The model under review builds one solid part; all positions refer to its coordinate system, in mm. A direction names the side the tool comes from. Coordinates: 2 decimals unless noted, no trailing zeros. Order: outer loops, then holes, each group sorted by start corner. A loop starts at its lowest first (then second) coordinate and runs counter-clockwise, first axis right, second up.
Autodesk Inventor part; units mm, degrees
ref_plane "YZ Plane" through (0, 0, 0) normal (1, 0, 0) x (0, 1, 0)
ref_plane "XZ Plane" through (0, 0, 0) normal (0, 1, 0) x (-1, 0, 0)
ref_plane "XY Plane" through (0, 0, 0) normal (0, 0, 1) x (1, 0, 0)
sketch "sketch" plane through (0, 0, 0) normal (0, 0, 1) x (1, 0, 0)
  line L0 (-10.4, 0) -> (62.4, 0) construction
  line L1 (0, -8.8) -> (0, 31.8) construction
  line L2 (0, 26) -> (52, 26)
  line L3 (52, 26) -> (52, 0)
  line L4 (52, 0) -> (0, 0)
  line L5 (0, 0) -> (0, 26)
  circle A0 centre (3.5, 19) radius 1.5
  circle A1 centre (3.5, 10) radius 1.5
  circle A2 centre (48.5, 19) radius 1.5
  circle A3 centre (48.5, 10) radius 1.5
  line L6 (10, 23) -> (42, 23)
  line L7 (42, 23) -> (42, 0)
  line L8 (42, 0) -> (10, 0)
  line L9 (10, 0) -> (10, 23)
  line L10 (0, 0) -> (52, 0)
  line L11 (52, 0) -> (52, -3)
  line L12 (52, -3) -> (0, -3)
  line L13 (0, -3) -> (0, 0)
  line L14 (7, 23) -> (10, 23)
  line L15 (10, 23) -> (10, 0)
  line L16 (10, 0) -> (7, 0)
  line L17 (7, 0) -> (7, 23)
  line L18 (42, 23) -> (45, 23)
  line L19 (45, 23) -> (45, 0)
  line L20 (45, 0) -> (42, 0)
  line L21 (42, 0) -> (42, 23)
  line L22 (0, 23) -> (7, 23)
  line L23 (45, 23) -> (52, 23)
  line L24 (7, 26) -> (7, 22.7671)
  line L25 (45, 26) -> (45, 23)
  line L26 (7, 0) -> (7, -3)
  line L27 (45, 0) -> (45, -3)
  point P0 (52, 0)
  dimension "d0" = 26
  dimension "d1" = 52
  dimension "d2" = 3
  dimension "d3" = 3
  dimension "d4" = 3
  dimension "d5" = 3
  dimension "d6" = 3.5
  dimension "d7" = 3.5
  dimension "d8" = 3.5
  dimension "d10" = 7
  dimension "d11" = 7
  dimension "d12" = 10
  dimension "d13" = 10
  dimension "d14" = 3
  dimension "d15" = 10
  dimension "d16" = 10
  dimension "d17" = 3
  dimension "d18" = 3
  dimension "d19" = 3
  dimension "d20" = 3.5
extrude "body" add sketch "sketch" along normal blind 50 contours L2 L25 L18 L6 L14 L24 | L14 L9 L4 L17 | L19 L4 L7 L18 | L4 L27 L12 L26
extrude "bolt" add sketch "sketch" along normal blind 1.5 contours L2 L24 L22 L5 | L22 L17 L4 L5 | L2 L3 L23 L25 | L4 L26 L12 L13 | L23 L3 L4 L19 | L4 L11 L12 L27
equation "\"d3\" = d2"
equation "\"d4\" = d2"
equation "\"d5\" = d2"
equation "\"d7\" = d6"
equation "\"d8\" = d6"
equation "\"d11\" = d10"
equation "\"d13\" = d12"
properties part number "battery"
(1) Consider section D-D (y = 19). Give the boundary of the cut face in (x, z), then the cut area to 3 significant figures.
(2) Consider section A-A (y = 16). Give the boundary of the cut face in (x, z), then the cut area to 3 significant figures.
(3) The part is to be moulded in two halves that separate along Y. For faces 1 (the face through (26, 0, 25)), 2 (the face through (45, 12, 25)), 3 (the face through (26, 26, 25)), say which applies: +Y half, -Y half, draft (parallel to the pull), parting line (faces both ways), or undercut.
(4) Tool access review of faces 4 (the face through (7, 12, 25)), 5 (the face through (48, 12, 1.5)), 6 (the face through (10, 11, 25)), 7 (the face through (26, -1, 50)): name each direction out of +Z, -Z, +X, -X, +Y, -Y from which nothing blocks a thin tool from reaching the whole face with its end or side.
(5) Wall thickness on line 1 (X direction, y = 11.5, z = 14); line 2 (Y direction, x = 25, z = 5.5); line 3 (Y direction, x = 3.5, z = 1.1): over which ranges is each line inside the solid? List them lowest first.
(6) Consider section C-C (z = 43.5). Give the boundary of the cut face in (x, y), then the cut area to 3 significant figures.
(7) Insertion check: pin 1 Ø4 at (y, z) = (14.5, 28.5) entering from -X; pin 2 Ø5.5 at (x, y) = (3, 9) entering from +Z; pin 3 Ø14.5 at (y, z) = (4.5, 21.5) entering from +X. Each pin has a flat end and moves straight along its axis. Give the tip position at first contact, or say it passes through.
(8) Consider section B-B (x = 48.5). Give the boundary of the cut face in (y, z).
Findings:
1. outline: (0, 0) - (2, 0) - (2, 1.5) - (0, 1.5) - close; (5, 0) - (10, 0) - (10, 50) - (7, 50) - (7, 1.5) - (5, 1.5) - close; (42, 0) - (47, 0) - (47, 1.5) - (45, 1.5) - (45, 50) - (42, 50) - close; (50, 0) - (52, 0) - (52, 1.5) - (50, 1.5) - close
1. area: 312 mm2
2. outline: (0, 0) - (10, 0) - (10, 50) - (7, 50) - (7, 1.5) - (0, 1.5) - close; (42, 0) - (52, 0) - (52, 1.5) - (45, 1.5) - (45, 50) - (42, 50) - close
2. area: 321 mm2
3. face 1: undercut
3. face 2: draft
3. face 3: +Y half
4. face 4: +Z, -X, +Y, -Y
4. face 5: +Z, +X, +Y, -Y
4. face 6: +Z, -Z
4. face 7: +Z, +X, -X, +Y, -Y
5. line 1: x = 7 to 10, 42 to 45
5. line 2: y = -3 to 0, 23 to 26
5. line 3: y = -3 to 8.5, 11.5 to 17.5, 20.5 to 26
6. outline: (7, -3) - (45, -3) - (45, 26) - (7, 26) - close; hole (10, 0) - (42, 0) - (42, 23) - (10, 23) - close
6. area: 366 mm2
7. pin 1: stops at x = 7
7. pin 2: stops at z = 1.5
7. pin 3: stops at x = 45
8. outline: (-3, 0) - (8.5, 0) - (8.5, 1.5) - (-3, 1.5) - close; (11.5, 0) - (17.5, 0) - (17.5, 1.5) - (11.5, 1.5) - close; (20.5, 0) - (26, 0) - (26, 1.5) - (20.5, 1.5) - close
